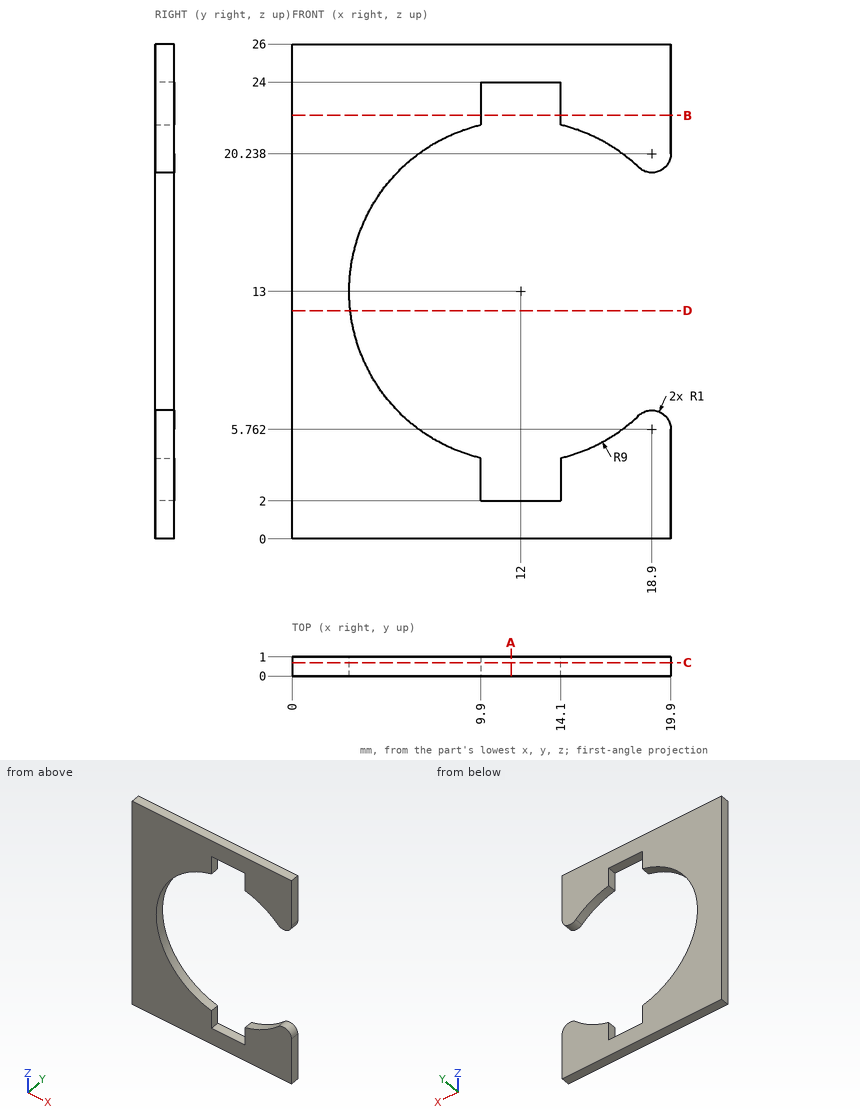
Could you check a few things on this drawing? It's one solid part, dimensions in mm from its lowest x, y, z. Coordinates: 2 decimals unless noted, no trailing zeros. Order: outer loops, then holes, each group sorted by start corner. A loop starts at its lowest first (then second) coordinate and runs counter-clockwise, first axis right, second up. Notation, with made-up numbers: (0, 34) -> (5, 34) arc R9 ccw to (5, 51) -> close; hole circle Ø8 at (46.25, -15). An arc over 180 degrees is marked (long way). One line per item, written item: value. Start each with the question number.
1) Imagine slicing it at D-D on z = 12. List the corners of the cut face in (x, y) for me.
2) Imagine slicing it at C-C on y = 0.7. List the corners of the cut face in (x, z) for me, plus the area to 3 significant figures.
3) Imagine slicing it at A-A on x = 11.5. List the corners of the cut face in (y, z) for me.
4) If I drill on L1, parallel to X at y = 0.4, z = 22; L2, parallel to Z at x = 13.5, y = 0.95; L3, parallel to Z at x = 15.5, y = 0.45, over which ranges is the centre line in solid material (lowest first)? Write a range as [from, to].
5) Imagine slicing it at B-B on z = 22.25. List the corners of the cut face in (x, y) for me.
Answer list:
1. outline: (0, 0) -> (3.06, 0) -> (3.06, 1) -> (0, 1) -> close
2. outline: (0, 0) -> (19.9, 0) -> (19.9, 5.76) arc R1 ccw to (18.21, 6.49) arc R9 cw to (14.1, 4.25) -> (14.1, 2) -> (9.9, 2) -> (9.9, 4.25) arc R9 cw to (9.9, 21.75) -> (9.9, 24) -> (14.1, 24) -> (14.1, 21.75) arc R9 cw to (18.21, 19.51) arc R1 ccw to (19.9, 20.24) -> (19.9, 26) -> (0, 26) -> close
2. area: 249 mm2
3. outline: (0, 0) -> (1, 0) -> (1, 2) -> (0, 2) -> close; (0, 24) -> (1, 24) -> (1, 26) -> (0, 26) -> close
4. L1: x = [0, 9.9], [14.1, 19.9]
4. L2: z = [0, 2], [24, 26]
4. L3: z = [0, 4.71], [21.29, 26]
5. outline: (0, 0) -> (9.9, 0) -> (9.9, 1) -> (0, 1) -> close; (14.1, 0) -> (19.9, 0) -> (19.9, 1) -> (14.1, 1) -> close
